```python
from build123d import *

# Parameters (mm, degrees)
ESQUISSE1_W        = 17.426618769
ESQUISSE1_H        = 9.816495883
BOSS_EXTRU_2_DEPTH = 5


with BuildPart() as part:
    # Esquisse1 → Boss.-Extru.2 (new body)
    with BuildSketch(Plane.XY):
        Polygon((-179.357380563, 206.271549111), (-179.357380563, 47.351549111), (-167.551475198, 47.351549111), (-167.551475198, 52.351549111), (-170.511475198, 52.351549111), (-170.511475198, 62.351549111), (-160.511475198, 62.351549111), (-160.511475198, 52.351549111), (-163.351475198, 52.351549111), (-163.351475198, 47.351549111), (-161.517380563, 47.351549111), (-147.887380563, 47.351549111), (-147.887380563, 42.351549111), (-97.887380563, 42.351549111), (-97.887380563, 47.351549111), (-79.987380563, 47.351549111), (-73.667421864, 47.351549111), (-57.887380563, 47.351549111), (-57.887380563, 42.351549111), (-7.887380563, 42.351549111), (-7.887380563, 47.351549111), (7.492660738, 47.351549111), (7.492660738, 52.351549111), (4.652660738, 52.351549111), (4.652660738, 62.351549111), (14.652660738, 62.351549111), (14.652660738, 52.351549111), (11.692660738, 52.351549111), (11.692660738, 47.351549111), (18.012619437, 47.351549111), (23.582619437, 47.351549111), (23.582619437, 206.271549111), (-7.887380563, 206.271549111), (-7.887380563, 211.271549111), (-57.887380563, 211.271549111), (-57.887380563, 206.271549111), (-73.667421864, 206.271549111), (-75.787380563, 206.271549111), (-75.787380563, 201.271549111), (-72.887380563, 201.271549111), (-72.887380563, 191.271549111), (-82.887380563, 191.271549111), (-82.887380563, 201.271549111), (-79.987380563, 201.271549111), (-79.987380563, 206.271549111), (-97.887380563, 206.271549111), (-97.887380563, 211.271549111), (-147.887380563, 211.271549111), (-147.887380563, 206.271549111), align=None)
        with BuildLine():
            Line((-87.92940723, 60.351549111), (-87.92940723, 87.351549111))
            ThreePointArc((-87.92940723, 87.351549111), (-77.92940723, 97.351549111), (-67.92940723, 87.351549111))
            Line((-67.92940723, 87.351549111), (-67.92940723, 60.351549111))
            ThreePointArc((-67.92940723, 60.351549111), (-77.92940723, 50.351549111), (-87.92940723, 60.351549111))
        make_face(mode=Mode.SUBTRACT)
        with Locations((-6.955391392, 92.259797053)):
            Rectangle(ESQUISSE1_W, ESQUISSE1_H, mode=Mode.SUBTRACT)
        with Locations((-148.903423068, 92.259797053)):
            Rectangle(ESQUISSE1_W, ESQUISSE1_H, mode=Mode.SUBTRACT)
    extrude(amount=BOSS_EXTRU_2_DEPTH)


solid = part.part
```
Verification items for the finished model (mm, model axes). A direction names the side the tool comes from. Coordinates: 2 decimals unless noted, no trailing zeros. Write each loop counter-clockwise with the first axis right and the second up, starting at its lowest first coordinate (ties: lowest second). Pieces come first, ordered by that corner, then holes. Notation, with made-up numbers: (55.25, 89) - (102.25, 89) arc R22 ccw to (102.25, 127) - close; hole circle Ø7 at (-6.5, 57.5). An arc over 180 degrees is marked (long way). One line per question, with ' | ' between items. Start each with the question number.
1. Gauge pin test, flat ends, axial feed: P1, Ø1.5, axis at x = 13, z = 3, coming from the +Y side; P2, Ø2.5, axis at y = 208.5, z = 2.5, coming from the +X side; P3, Ø1.5, axis at x = -2.5, z = 3.5, coming from the -Y side. Record the tip position at first contact, or that the pin passes through.
2. Section check B-B (z = 1.7). Count the separate pieces of the cut face and the enclosed holes in it, plus the area to 3 significant figures.
3. Access from +Z, -Z, +X, -X, +Y, -Y to the whole of each face (thin tool, end or side, straight path). Record for faces 1 (the flat face through (8, 206.272, 2)), 2 (the flat face through (-160.511, 57, 2)), 3 (the flat face through (-79.987, 204, 2)).
4. Section check C-C (x = -92). Enter the section's corners in (y, z).
5. Section check A-A (x = -144.5). Enter the section's corners in (y, z).
6. Material ranges on line 1 along X through (y, z) = (75, 4.6); line 2 along Y through (x, z) = (-161.5, 0.85); line 3 along X through (y, z) = (200, 4.6), recorded low to high.
Computed values:
1) P1: y = 206.27 | P2: x = -7.89 | P3: y = 47.35
2) separate pieces: 1 | enclosed holes: 3 | area: 31,700 mm²
3) face 1: +Z, -Z, +X, +Y | face 2: +Z, -Z | face 3: +Z, -Z, +Y
4) outline: (47.35, 0) - (206.27, 0) - (206.27, 5) - (47.35, 5) - close
5) outline: (42.35, 0) - (87.35, 0) - (87.35, 5) - (42.35, 5) - close; (97.17, 0) - (211.27, 0) - (211.27, 5) - (97.17, 5) - close
6) line 1: -179.36 to -87.93, -67.93 to 23.58 | line 2: 47.35 to 52.35, 62.35 to 206.27 | line 3: -179.36 to -82.89, -72.89 to 23.58
